Work out the finished part from the listing and answer in its coordinate system (mm). Face numbers are marked on the shaded views. Give positions to 0.01 mm unless a question says otherwise; leave off trailing zeros. Write each loop counter-clockwise with the first axis right and the second up, starting at its lowest first coordinate (ties: lowest second). Pieces come first, ordered by that corner, then holes.
1) Find section B-B (x = 39.5). Determine the outline of the cut face in (y, z), plus the area to 3 significant figures.
2) Find section C-C (x = 56.5). Determine the outline of the cut face in (y, z), plus the area to 3 significant figures.
3) Straight lines are drawn through the part: probe 1 along Y at (x, z) = (23.5, -59); probe 2 along Y at (x, z) = (62.5, 2); probe 3 along X at (y, z) = (-2, -26). For each, find the intervals that lie inside material, in ascending order.
4) Find section A-A (z = 5). Determine the outline of the cut face in (x, y).
5) Determine the mould class of the marked faces 1 and 2 for opening direction X: pulls with the +X half, pulls with the -X half, needs draft (parallel to the pull), parting line crosses it, or undercut.
6) Given pin 1 Ø3 at (x, y) = (3, -2.5) entering from +Z; pin 2 Ø0.5 at (x, y) = (43.5, 0) entering from +Z; pin 3 Ø3 at (x, y) = (2, -3) entering from -Z; pin 4 Ø0.5 at (y, z) = (0, -48.5) entering from -X, each flat-ended and moving along its own axis, determine where each tip first touches the part or whether it passes through.
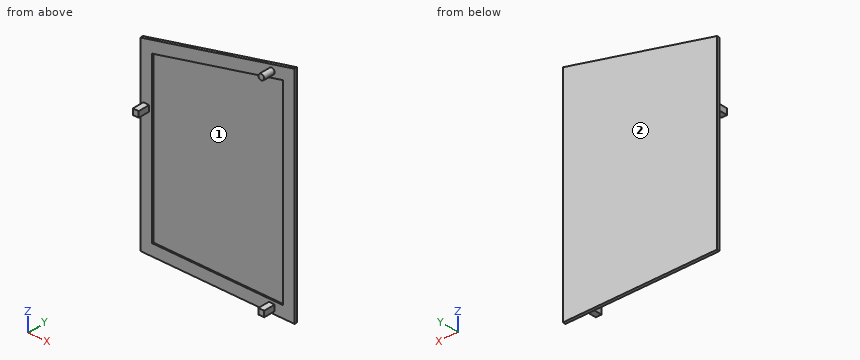
```python
from build123d import *

# Parameters (mm, degrees)
BOSS_EXTRUDE1_DEPTH = 1.25
SKETCH2_R           = 1.25
SKETCH2_W           = 2.5
SKETCH2_H           = 2.5
BOSS_EXTRUDE2_DEPTH = 5
CUT_EXTRUDE1_DEPTH  = 0.6


with BuildPart() as part:
    # Sketch1 → Boss-Extrude1 (new body)
    with BuildSketch(Plane(origin=(0, 0, 0), x_dir=(1, 0, 0), z_dir=(0, 1, 0))):
        Polygon((0, 0), (0, 80), (66.3, 80), (66.3, -15.623791318), align=None)
    extrude(amount=BOSS_EXTRUDE1_DEPTH)

    # Sketch2 → Boss-Extrude2 (add)
    with BuildSketch(Plane.XZ):
        with Locations(Location((56.5, 10.745914737, 0), (0, 0, 270))):
            Circle(SKETCH2_R)
        with Locations((56.5, -77.5)):
            Rectangle(SKETCH2_W, SKETCH2_H)
        with Locations((2.5, -25)):
            Rectangle(SKETCH2_W, SKETCH2_H)
    extrude(amount=BOSS_EXTRUDE2_DEPTH)

    # Sketch3 → Cut-Extrude1 (cut)
    with BuildSketch(Plane(origin=(0, 0, 0), x_dir=(-1, 0, 0), z_dir=(0, -1, 0))):
        Polygon((-61.3, 75), (-61.3, -9.308571388), (-5, 3.958690319), (-5, 75), align=None)
    extrude(amount=-CUT_EXTRUDE1_DEPTH, mode=Mode.SUBTRACT)


solid = part.part
```
Results:
1. outline: (0, -80) - (1.25, -80) - (1.25, 9.31) - (0, 9.31) - (0, 4.17) - (0.6, 4.17) - (0.6, -75) - (0, -75) - close
1. area: 64.1 mm2
2. outline: (-5, -78.75) - (0, -78.75) - (0, -80) - (1.25, -80) - (1.25, 13.31) - (0, 13.31) - (0, 12) - (-5, 12) - (-5, 9.5) - (0, 9.5) - (0, 8.18) - (0.6, 8.18) - (0.6, -75) - (0, -75) - (0, -76.25) - (-5, -76.25) - close
2. area: 91.7 mm2
3. probe 1: y = 0.6 to 1.25
3. probe 2: y = 0 to 1.25
3. probe 3: x = 1.25 to 3.75
4. outline: (21.22, 0) - (43.02, 0) - (43.02, 0.6) - (61.3, 0.6) - (61.3, 0) - (66.3, 0) - (66.3, 1.25) - (21.22, 1.25) - close
5. face 1: undercut
5. face 2: needs draft
6. pin 1: stops at z = -23.75
6. pin 2: stops at z = 10.31
6. pin 3: stops at z = -26.25
6. pin 4: stops at x = 0
